Input: dimensioned drawing with shaded views. Units: mm. Origin: part minimum x, y, z. A direction names the side the tool comes from. Round coordinates to 2 decimals unless told otherwise and drop trailing zeros. Loops run counter-clockwise (first coordinate to the right, second up) from the corner with the lowest first, then second, coordinate; pieces in that order, holes last.
1) First-contact query: pin 1 (12 mm diameter, centred on x = 37.5, z = 32.5, fed in from -Y); pin 2 (1 mm diameter, centred on x = 7.5, z = 46, fed in from -Y); pin 3 (5 mm diameter, centred on y = 27.5, z = 26.5, fed in from +X) (1 decimal); pin 4 (5 mm diameter, centred on x = 35, z = 42, fed in from +Y). Flat tips, straight axial feed; report the tip coordinate or a pass-through.
2) Access query for the marked faces 1 and 2. Directions: +Z, -Z, +X, -X, +Y, -Y. A direction counts if a zero-diameter tool reaches every point of the face in a straight line with its end or side. Return the directions, or none.
3) Section D-D, the plane x = 40.5. Return loops of the section in (y, z) (1 decimal), and give its area (3 significant figures).
4) Section A-A, the plane x = 13.5. Return loops of the section in (y, z), and give its area (3 significant figures).
5) Section C-C, the plane z = 21.5. Return loops of the section in (x, y) (1 decimal), and give its area (3 significant figures).
6) Section B-B, the plane y = 74.5. Return loops of the section in (x, z), and give its area (3 significant figures).
7) Ray query, line 1 along Y through (x, z) = (6.5, 55) (1 decimal); line 2 along Y through (x, z) = (8, 50) (1 decimal); line 3 along Y through (x, z) = (10, 46.5) (1 decimal). Return the intervals inside material, ascending.
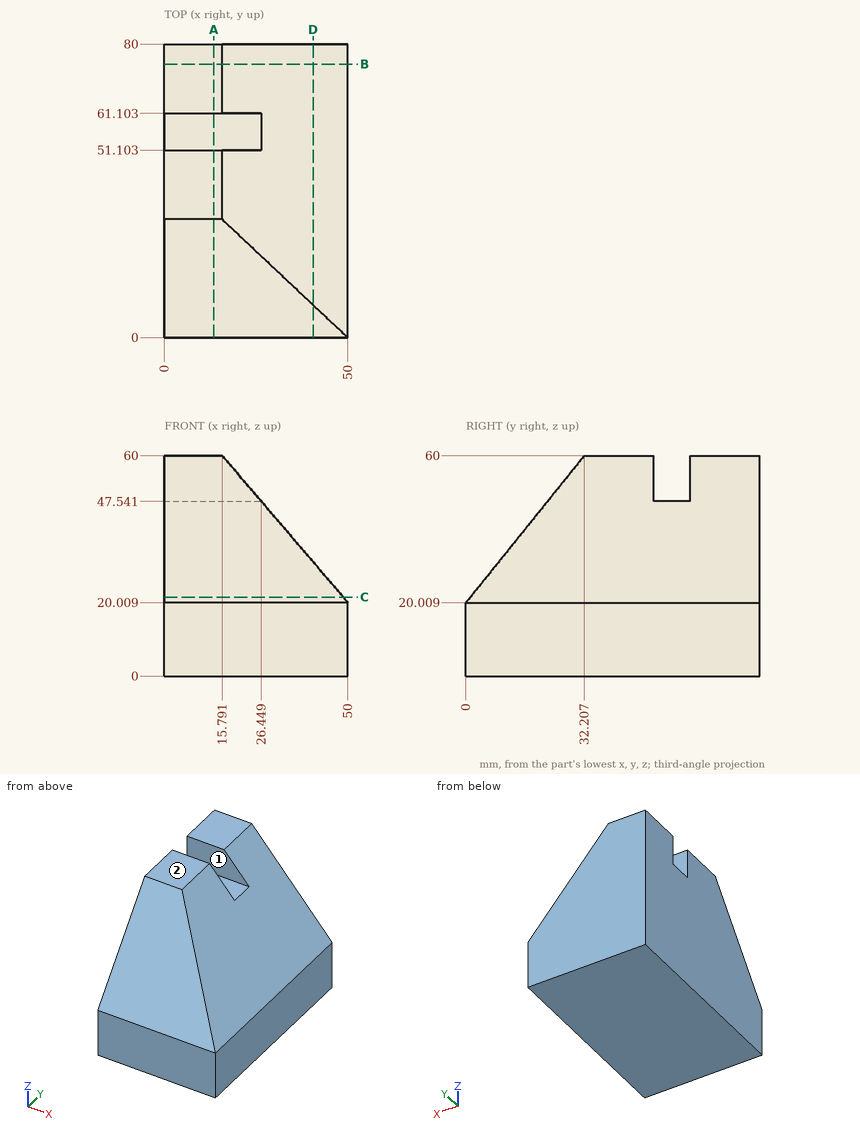
Final values:
1. pin 1: stops at y = 5.23
1. pin 2: stops at y = 20.53
1. pin 3: stops at x = 46.6
1. pin 4: passes through
2. face 1: +Z, +X, -X
2. face 2: +Z, +X, -X, +Y, -Y
3. outline: (0, 0) - (80, 0) - (80, 31.1) - (8.9, 31.1) - (0, 20) - close
3. area: 2,440 mm2
4. outline: (0, 0) - (80, 0) - (80, 60) - (61.1, 60) - (61.1, 47.54) - (51.1, 47.54) - (51.1, 60) - (32.21, 60) - (0, 20.01) - close
4. area: 4,030 mm2
5. outline: (0, 1.2) - (48.7, 1.2) - (48.7, 80) - (0, 80) - close
5. area: 3,840 mm2
6. outline: (0, 0) - (50, 0) - (50, 20.01) - (15.79, 60) - (0, 60) - close
6. area: 2,320 mm2
7. line 1: y = 28.2 to 51.1, 61.1 to 80
7. line 2: y = 24.2 to 51.1, 61.1 to 80
7. line 3: y = 21.3 to 80
